Could you check a few things on this model? Use its own coordinates, in mm. Face numbers are marked on the shaded views. A direction names the side the tool comes from. Give positions to 0.01 mm unless a question says otherwise; leave off trailing zeros. Order: outer loops, then holes, each group sorted by start corner. A loop starts at its lowest first (then second) coordinate and runs counter-clockwise, first axis right, second up. Notation, with made-up numbers: M 68,15 L 91,15 A25 cw 91,34 Z; hole C 38.5,87.5 d7. An arc over 180 degrees is marked long. Use a Markdown table: item, result. Add a question column.
```python
from build123d import *

# Parameters (mm, degrees)
F0_W     = 431.8
F0_H     = 203.2
F1_DEPTH = 355.6
F2_W     = 413.108602
F2_H     = 340.378207
F3_DEPTH = 195.58
F4_R     = 25.4
F5_DEPTH = 20.066
F6_W     = 43.054437
F6_H     = 10.763585
F7_DEPTH = 195.581


with BuildPart() as f1:
    # F0 (on Front) → F1 (new body)
    with BuildSketch(Plane.XZ):
        Rectangle(F0_W, F0_H)
    extrude(amount=F1_DEPTH)

    # F2 (on face) → F3 (cut)
    with BuildSketch(Plane.XY.offset(101.6)):
        with Locations((0.110827, -177.696624)):
            Rectangle(F2_W, F2_H)
    extrude(amount=-F3_DEPTH, mode=Mode.SUBTRACT)

    # F4 (on face) → F5 (join)
    with BuildSketch(Plane.XZ.offset(355.6)):
        with Locations((0, 48.113549)):
            Circle(F4_R)
    extrude(amount=F5_DEPTH)

    # F6 (on face) → F7 (cut, through all)
    with BuildSketch(Plane.XY.offset(-93.98)):
        with Locations((-0.160011, -367.300331)):
            Rectangle(F6_W, F6_H)
    extrude(amount=F7_DEPTH, mode=Mode.SUBTRACT)


solid = f1.part
```
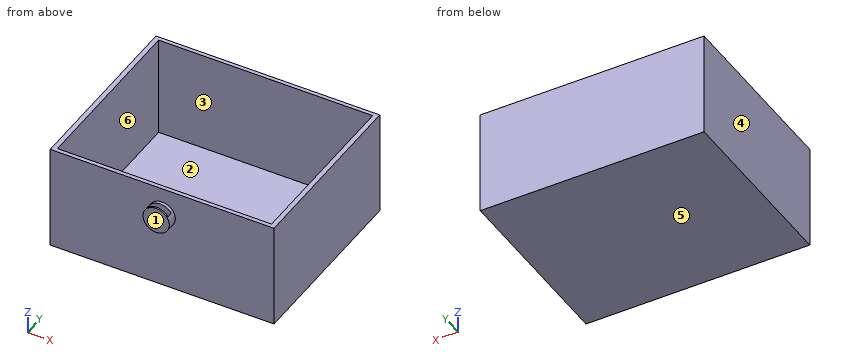
1) Suppose I cut it at C-C on x = -80. Please give me the cut outline in (y, z), and give its area (3 significant figures).
2) Suppose I cut it at A-A on x = 0. Please give me the cut outline in (y, z).
3) Please list where these lines run through material, in increasing order: line 1 (Y direction, x = 135.5, z = 32); line 2 (X direction, y = -303, z = -41.5); line 3 (Z direction, x = -148.5, y = -239.5). Write a range as from..to.
4) We'd pull the mould along X, two halves only. Please class the marked faces 3, 4, 5 and 6: pulls with the +X half, pulls with the -X half, needs draft (parallel to the pull), parting line crosses it, or undercut.
5) Suppose I cut it at B-B on z = -41. Please give me the cut outline in (x, y), and give its area (3 significant figures).
6) For pin 1 (2 mm diameter, centred on x = 42.5, y = -54, fed in from +Z); pin 2 (8.5 mm diameter, centred on y = -365, z = 47.5, fed in from +X); pin 3 (12 mm diameter, centred on x = 36.5, z = -76.5, fed in from -Y), each with a flat end and sliding along its axis, tell me the tip position at first contact or that it passes through.
7) For the marked faces 1 and 2, which set-ups out of +Z, -Z, +X, -X, +Y, -Y let a thin tool reach every point of the face, with its end or its side?
Values found:
| question | item | result |
|---|---|---|
| 1 | outline | M -355.6,-101.6 L 0,-101.6 L 0,101.6 L -7.51,101.6 L -7.51,-93.98 L -347.89,-93.98 L -347.89,101.6 L -355.6,101.6 Z |
| 1 | area | 5,690 mm^2 |
| 2 | outline | M -375.67,22.71 L -372.68,22.71 L -372.68,73.51 L -375.67,73.51 Z; M -361.92,22.71 L -355.6,22.71 L -355.6,-101.6 L 0,-101.6 L 0,101.6 L -7.51,101.6 L -7.51,-93.98 L -347.89,-93.98 L -347.89,101.6 L -355.6,101.6 L -355.6,73.51 L -361.92,73.51 Z |
| 3 | line 1 | y = -355.6..-347.89, -7.51..0 |
| 3 | line 2 | x = -215.9..-206.44, 206.67..215.9 |
| 3 | line 3 | z = -101.6..-93.98 |
| 4 | face 3 | undercut |
| 4 | face 4 | pulls with the -X half |
| 4 | face 5 | needs draft |
| 4 | face 6 | undercut |
| 5 | outline | M -215.9,-355.6 L 215.9,-355.6 L 215.9,0 L -215.9,0 Z; hole M -206.44,-347.89 L 206.67,-347.89 L 206.67,-7.51 L -206.44,-7.51 Z |
| 5 | area | 12,900 mm^2 |
| 6 | pin 1 | stops at z = -93.98 |
| 6 | pin 2 | stops at x = 25.4 |
| 6 | pin 3 | stops at y = -355.6 |
| 7 | face 1 | +Z, -Z, +X, -X, -Y |
| 7 | face 2 | +Z |
